Check sheet for the modelled part. Datum: model origin and axes. Units: mm. A direction names the side the tool comes from. Give positions to 0.01 mm unless a question says otherwise; leave off trailing zeros. Write each loop counter-clockwise with the first axis right and the second up, starting at its lowest first coordinate (ties: lowest second). Pieces come first, ordered by that corner, then holes. Notation, with made-up numbers: M -11,27.5 L -2,27.5 A24 ccw -2,54.5 Z; hole C 13,-25 d7. An arc over 180 degrees is marked long. One line per item, written item: value. Start each with the question number.
from build123d import *

# Parameters (mm, degrees)
SKETCH1_W           = 143
SKETCH1_H           = 143
SKETCH1_W_2         = 98
SKETCH1_H_2         = 98
BOSS_EXTRUDE1_DEPTH = 3
SKETCH2_W           = 143
SKETCH2_H           = 143
SKETCH2_W_2         = 141
SKETCH2_H_2         = 141
BOSS_EXTRUDE2_DEPTH = 35
SKETCH3_W           = 21.5
SKETCH3_H           = 21.5
BOSS_EXTRUDE3_DEPTH = 4
SKETCH4_W           = 9.937019223
SKETCH4_H           = 9.54986263
CUT_EXTRUDE1_DEPTH  = 4


with BuildPart() as part:
    # Sketch1 → Boss-Extrude1 (new body)
    with BuildSketch(Plane.XY):
        Rectangle(SKETCH1_W, SKETCH1_H)
        Rectangle(SKETCH1_W_2, SKETCH1_H_2, mode=Mode.SUBTRACT)
    extrude(amount=BOSS_EXTRUDE1_DEPTH)

    # Sketch2 → Boss-Extrude2 (add)
    with BuildSketch(Plane(origin=(0, 0, 0), x_dir=(-1, 0, 0), z_dir=(0, 0, -1))):
        Rectangle(SKETCH2_W, SKETCH2_H)
        Rectangle(SKETCH2_W_2, SKETCH2_H_2, mode=Mode.SUBTRACT)
    extrude(amount=BOSS_EXTRUDE2_DEPTH)

    # Sketch3 → Boss-Extrude3 (add)
    with BuildSketch(Plane(origin=(0, 0, 0), x_dir=(-1, 0, 0), z_dir=(0, 0, -1))):
        with Locations((-59.75, 59.75)):
            Rectangle(SKETCH3_W, SKETCH3_H)
        with Locations((-59.75, -59.75)):
            Rectangle(SKETCH3_W, SKETCH3_H)
        with Locations((59.75, -59.75)):
            Rectangle(SKETCH3_W, SKETCH3_H)
        with Locations((59.75, 59.75)):
            Rectangle(SKETCH3_W, SKETCH3_H)
    extrude(amount=BOSS_EXTRUDE3_DEPTH)

    # Sketch4 → Cut-Extrude1 (cut)
    with BuildSketch(Plane(origin=(0, 71.5, 0), x_dir=(1, 0, 0), z_dir=(0, 1, 0))):
        with Locations((-45.619951888, 12.228924985)):
            Rectangle(SKETCH4_W, SKETCH4_H)
    extrude(amount=-CUT_EXTRUDE1_DEPTH, mode=Mode.SUBTRACT)


solid = part.part
1) Tool access check on faces 4 (the flat face through (71.5, -1, -16)), 5 (the flat face through (-60, 1, 0)). Record the directions out of +Z, -Z, +X, -X, +Y, -Y that give a thin tool (end or side, any length) a straight path to the whole face; none if there is none.
2) Draft check along Y on faces 1 (the flat face through (1, -71.5, -16)), 2 (the flat face through (-60, 60, -4)), 3 (the flat face through (63, 1, 3)). Enter one of: released by +Y, released by -Y, zero draft, split by the parting line, or undercut.
3) Gauge pin test, flat ends, axial feed: pin 1 (17 mm diameter, centred on x = -2, y = -61.5, fed in from -Z); pin 2 (6.5 mm diameter, centred on x = -64, y = 57.5, fed in from -Z). Record the tip position at first contact, or that the pin passes through.
4) Cross-section at A-A (y = -25). Record the boundary of the cut face in (x, z), plus the area to 3 significant figures.
5) Cross-section at D-D (x = 62.5). Record the boundary of the cut face in (y, z), plus the area to 3 significant figures.
6) Cross-section at C-C (z = -20). Record the boundary of the cut face in (x, y).
7) Material ranges on L1, parallel to X at y = 2, z = -21; L2, parallel to Y at x = -61, z = -3, recorded low to high. Write a range as from..to.
Data:
1. face 4: +Z, -Z, +X, +Y, -Y
1. face 5: -Z
2. face 1: released by -Y
2. face 2: undercut
2. face 3: zero draft
3. pin 1: stops at z = 0
3. pin 2: stops at z = -4
4. outline: M -71.5,-35 L -70.5,-35 L -70.5,0 L -49,0 L -49,3 L -71.5,3 Z; M 49,0 L 70.5,0 L 70.5,-35 L 71.5,-35 L 71.5,3 L 49,3 Z
4. area: 205 mm2
5. outline: M -71.5,-35 L -70.5,-35 L -70.5,-4 L -49,-4 L -49,0 L 49,0 L 49,-4 L 70.5,-4 L 70.5,-35 L 71.5,-35 L 71.5,3 L -71.5,3 Z
5. area: 671 mm2
6. outline: M -71.5,-71.5 L 71.5,-71.5 L 71.5,71.5 L -71.5,71.5 Z; hole M -70.5,-70.5 L 70.5,-70.5 L 70.5,70.5 L -70.5,70.5 Z
7. L1: x = -71.5..-70.5, 70.5..71.5
7. L2: y = -71.5..-49, 49..71.5
